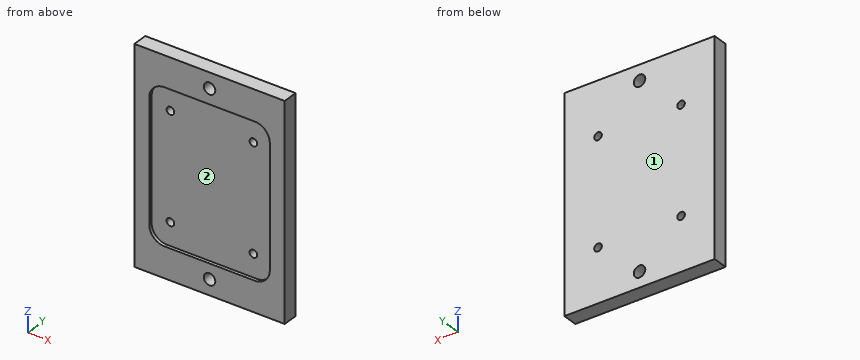
from build123d import *

# Parameters (mm, degrees)
SKETCH2_W           = 63.25
SKETCH2_H           = 89.08
BOSS_EXTRUDE1_DEPTH = 6.32
SKETCH3_R           = 2.415
CUT_EXTRUDE1_DEPTH  = 6.32
SKETCH4_R           = 2.415
CUT_EXTRUDE2_DEPTH  = 6.32
SKETCH5_W           = 50.72
SKETCH5_H           = 63.55
CUT_EXTRUDE3_DEPTH  = 1.37
FILLET1_R           = 6.35
SKETCH7_R           = 1.6
CUT_EXTRUDE4_DEPTH  = 5.95


with BuildPart() as part:
    # Sketch2 → Boss-Extrude1 (new body)
    with BuildSketch(Plane(origin=(0, 0, 0), x_dir=(1, 0, 0), z_dir=(0, 1, 0))):
        with Locations((31.625, 44.54)):
            Rectangle(SKETCH2_W, SKETCH2_H)
    extrude(amount=BOSS_EXTRUDE1_DEPTH)

    # Sketch3 → Cut-Extrude1 (cut)
    with BuildSketch(Plane(origin=(0, 0, 0), x_dir=(-1, 0, 0), z_dir=(0, -1, 0))):
        with Locations((-31.625, 82.65)):
            Circle(SKETCH3_R)
    extrude(amount=-CUT_EXTRUDE1_DEPTH, mode=Mode.SUBTRACT)

    # Sketch4 → Cut-Extrude2 (cut)
    with BuildSketch(Plane(origin=(0, 0, 0), x_dir=(-1, 0, 0), z_dir=(0, -1, 0))):
        with Locations((-31.625, 6.43)):
            Circle(SKETCH4_R)
    extrude(amount=-CUT_EXTRUDE2_DEPTH, mode=Mode.SUBTRACT)

    # Sketch5 → Cut-Extrude3 (cut)
    with BuildSketch(Plane(origin=(0, 0, 0), x_dir=(-1, 0, 0), z_dir=(0, -1, 0))):
        with Locations((-31.625, 44.54)):
            Rectangle(SKETCH5_W, SKETCH5_H)
    extrude(amount=-CUT_EXTRUDE3_DEPTH, mode=Mode.SUBTRACT)

    # Fillet1
    fillet1_edges = [part.edges().sort_by_distance(p)[0] for p in [
        (56.985, 0.685, -12.765),
        (56.985, 0.685, -76.315),
        (6.265, 0.685, -76.315),
        (6.265, 0.685, -12.765),
    ]]
    fillet(fillet1_edges, radius=FILLET1_R)

    # Sketch7 → Cut-Extrude4 (cut, through all)
    with BuildSketch(Plane(origin=(0, 1.37, 0), x_dir=(-1, 0, 0), z_dir=(0, -1, 0))):
        with Locations((-49.09, 22.315)):
            Circle(SKETCH7_R)
        with Locations((-49.09, 66.765)):
            Circle(SKETCH7_R)
        with Locations((-14.16, 66.765)):
            Circle(SKETCH7_R)
        with Locations((-14.16, 22.315)):
            Circle(SKETCH7_R)
    extrude(amount=-CUT_EXTRUDE4_DEPTH, mode=Mode.SUBTRACT)


solid = part.part
Source: CAD feature listing. Evaluate the final solid. Frame: model axes, mm. Face numbers are marked on the shaded views. Give positions to 0.01 mm unless a question says otherwise; leave off trailing zeros. Write each loop counter-clockwise with the first axis right and the second up, starting at its lowest first coordinate (ties: lowest second). Pieces come first, ordered by that corner, then holes. Notation, with made-up numbers: M -12.75,41.25 L 21.25,41.25 A26 ccw 21.25,69.25 Z; hole C -8,-13 d5. An arc over 180 degrees is marked long. Return JSON: item names as keys, results as strings. Group by question number.
1) Draft query along Z for the marked faces 1 and 2. Return one class per face: released by +Z, released by -Z, zero draft, split by the parting line, or undercut.
2) Ray query, L1, parallel to Z at x = 14.16, y = 4.35 (3 decimals); L2, parallel to X at y = 2, z = -6.43; L3, parallel to Z at x = 48.5, y = 4.5. Return the intervals inside material, ascending.
3) Cut plane D-D, the plane x = 32.5. Output: boundary loops of the cut face in (y, z) (3 decimals), then the cut area to 3 significant figures.
4) Cut plane A-A, the plane x = 49.09. Output: boundary loops of the cut face in (y, z) (3 decimals).
5) First-contact query: pin 1 Ø3.5 at (x, z) = (14.16, -22.315) entering from -Y; pin 2 Ø1.9 at (x, z) = (49.09, -66.765) entering from +Y. Flat tips, straight axial feed; report the tip coordinate or a pass-through.
6) Cut plane C-C, the plane z = -58.5. Output: boundary loops of the cut face in (x, y) (3 decimals), then the cut area to 3 significant figures.
7) Cut plane B-B, the plane z = -82.65. Output: boundary loops of the cut face in (x, y).
Data:
{
 "1": {"face 1": "zero draft", "face 2": "undercut"},
 "2": {"L1": "z = -89.08 to -68.365, -65.165 to -23.915, -20.715 to 0", "L2": "x = 0 to 29.21, 34.04 to 63.25", "L3": "z = -89.08 to -68.25, -65.28 to -23.8, -20.83 to 0"},
 "3": {"outline": "M 0,-89.08 L 6.32,-89.08 L 6.32,-84.901 L 0,-84.901 Z; M 0,-80.399 L 6.32,-80.399 L 6.32,-8.681 L 0,-8.681 L 0,-12.765 L 1.37,-12.765 L 1.37,-76.315 L 0,-76.315 Z; M 0,-4.179 L 6.32,-4.179 L 6.32,0 L 0,0 Z", "area": "419 mm²"},
 "4": {"outline": "M 0,-89.08 L 6.32,-89.08 L 6.32,-68.365 L 1.37,-68.365 L 1.37,-76.315 L 0,-76.315 Z; M 0,-12.765 L 1.37,-12.765 L 1.37,-20.715 L 6.32,-20.715 L 6.32,0 L 0,0 Z; M 1.37,-65.165 L 6.32,-65.165 L 6.32,-23.915 L 1.37,-23.915 Z"},
 "5": {"pin 1": "stops at y = 1.37", "pin 2": "passes through"},
 "6": {"outline": "M 0,0 L 6.265,0 L 6.265,1.37 L 56.985,1.37 L 56.985,0 L 63.25,0 L 63.25,6.32 L 0,6.32 Z", "area": "330 mm²"},
 "7": {"outline": "M 0,0 L 29.21,0 L 29.21,6.32 L 0,6.32 Z; M 34.04,0 L 63.25,0 L 63.25,6.32 L 34.04,6.32 Z"}
}
